Input: part model. Units: mm. Frame: model coordinates. A direction names the side the tool comes from. Coordinates: 2 decimals unless noted, no trailing zeros. Loops run counter-clockwise (first coordinate to the right, second up) from the corner with the lowest first, then second, coordinate; pieces in that order, holes last. Notation, with made-up numbers: M -11,75 L 34,75 A24 cw 34,110 Z; hole C 81,48 d4. An arc over 180 degrees is marked long. Use a Markdown table: item, result. Add a question column.
1. Section C-C on y = 0. Output: boundary loops of the cut face in (x, z).
2. Draft query along X for faces 1 (the cylindrical face through (-1.144, 8.713, 34.15)), 2 (the cylindrical face through (-2.25, 17.136, 30.206)), 3 (the flat face through (-0.7, 6.646, 7.809)). Return one class per face: +X half, -X half, draft (parallel to the pull), parting line (faces both ways), or undercut.
3. Section A-A on z = 36.5. Output: boundary loops of the cut face in (x, y).
4. Set-up query: faces 4 (the flat face through (50, 9, 7)), 5 (the flat face through (-8, 4, 50)), 6 (the flat face through (45.567, 8, 8)). Return all of +Z, -Z, +X, -X, +Y, -Y with unobstructed straight access to the full face (end or side cutting, diameter ignored); none if empty.
5. Section B-B on x = -27. Output: boundary loops of the cut face in (y, z).
6. Pin query (flat end, axial travel): pin 1 (14 mm diameter, centred on x = 0, y = 0, fed in from -Z); pin 2 (1.5 mm diameter, centred on x = 13, z = 28.5, fed in from -Y); pin 3 (12 mm diameter, centred on x = 22, z = 7, fed in from +Y). Return the tip coordinate at first contact, or that it passes through.
7. Section D-D on z = -24. Output: boundary loops of the cut face in (x, y), then the cut area to 3 significant figures.
8. Line query: L1, parallel to X at y = 0, z = 20.5; L2, parallel to Y at x = 0, z = 35; L3, parallel to Y at x = 0, z = 31. Output: solid intervals per line, ascending. Write a range as [from, to].
```python
from build123d import *

# Parameters (mm, degrees)
F0_R     = 17.283022434
F1_DEPTH = 50
F2_R     = 8.7881586796
F3_DEPTH = 50
F5_DEPTH = 20
F7_W     = 100
F7_H     = 117.4868202522
F8_DEPTH = 2


with BuildPart() as f1:
    # F0 (on Top) → F1 (new body)
    with BuildSketch(Plane.XY):
        Circle(F0_R)
    extrude(amount=F1_DEPTH)

    # F2 (on face) → F3 (cut)
    with BuildSketch(Plane.XY.offset(50)):
        Circle(F2_R)
    extrude(amount=-F3_DEPTH, mode=Mode.SUBTRACT)

    # F4 (on Right) → F5 (cut, symmetric)
    with BuildSketch(Plane.YZ):
        Polygon((-17.283022434, 34.5660448679), (-17.283022434, 0), (17.283022434, 0), align=None)
    extrude(amount=F5_DEPTH, both=True, mode=Mode.SUBTRACT)

    # F7 (on offset) → F8 (join)
    with BuildSketch(Plane(origin=(0, 8.641511217, 8.641511217), x_dir=(1, 0, 0), z_dir=(0, -0.7071067812, -0.7071067812))):
        Rectangle(F7_W, F7_H)
        with BuildLine():
            ThreePointArc((38.4038900758, -0.7964591027), (28.4677323699, 0), (38.4038900758, 0.7964591027))
            Line((38.4038900758, 0.7964591027), (45.567390877, 0.7964591027))
            Line((45.567390877, 0.7964591027), (45.567390877, -0.7964591027))
            Line((45.567390877, -0.7964591027), (38.4038900758, -0.7964591027))
        make_face(mode=Mode.SUBTRACT)
    extrude(amount=F8_DEPTH)


solid = f1.part
```
Answers below:
| question | item | result |
|---|---|---|
| 1 | outline | M -50,14.45 L 50,14.45 L 50,17.28 L 17.28,17.28 L 17.28,50 L 8.79,50 L 8.79,17.28 L -8.79,17.28 L -8.79,50 L -17.28,50 L -17.28,17.28 L -50,17.28 Z |
| 2 | face 1 | undercut |
| 2 | face 2 | parting line |
| 2 | face 3 | draft |
| 3 | outline | M -50,-22.05 L 50,-22.05 L 50,-19.22 L -50,-19.22 Z; C 0,0 d34.57; hole C 0,0 d17.58 |
| 4 | face 4 | +Z, -Z, +X, +Y, -Y |
| 4 | face 5 | +Z, +X, -X, +Y |
| 4 | face 6 | none |
| 5 | outline | M -34.31,48.77 L 48.77,-34.31 L 50.18,-32.9 L -32.9,50.18 Z |
| 6 | pin 1 | stops at z = 7.45 |
| 6 | pin 2 | stops at y = -14.8 |
| 6 | pin 3 | stops at y = 16.28 |
| 7 | outline | M -50,38.45 L 50,38.45 L 50,41.28 L -50,41.28 Z |
| 7 | area | 283 mm² |
| 8 | L1 | x = [-17.28, -8.79], [8.79, 17.28] |
| 8 | L2 | y = [-20.55, -17.72], [-17.28, -8.79], [8.79, 17.28] |
| 8 | L3 | y = [-16.55, -8.79], [8.79, 17.28] |
